Read the model definition and answer for the solid it produces. Units are mm, in the model's axes. A direction names the side the tool comes from. Coordinates: 2 decimals unless noted, no trailing zeros. Order: outer loops, then holes, each group sorted by start corner. A loop starts at its lowest first (then second) coordinate and runs counter-clockwise, first axis right, second up. Notation, with made-up numbers: M 56,68.25 L 75,68.25 A20 ccw 75,88.25 Z; hole C 80.25,87.25 d9. An arc over 180 degrees is marked long. Put each result on its own line as item: value.
from build123d import *

# Parameters (mm, degrees)
CUT_EXTRUDE1_REACH = 68.227
SKETCH4_W          = 8
SKETCH4_H          = 13


with BuildPart() as part:
    # Sketch1 → Revolve1 (revolve)
    with BuildSketch(Plane.XY, mode=Mode.PRIVATE) as revolve1_sk:
        Polygon((0, 25), (0, 7.5), (-40, 7.5), (-40, 6.5), (19, 6.5), (19, 12), (56, 12), (56, 14), (6, 14), (6, 25), align=None)
    revolve(revolve1_sk.sketch.rotate(Axis((-64.900117457, 0, 0), (1, 0, 0)), 180), axis=Axis((-64.900117457, 0, 0), (1, 0, 0)))

    # Sketch4 → Cut-Extrude1 (cut, up to next)
    with BuildSketch(Plane(origin=(0, 0, 0), x_dir=(1, 0, 0), z_dir=(0, 1, 0)), mode=Mode.PRIVATE) as cut_extrude1_sk1:
        with Locations((15, 0)):
            Rectangle(SKETCH4_W, SKETCH4_H)
    cut_extrude1_tool1 = extrude(cut_extrude1_sk1.sketch, amount=-CUT_EXTRUDE1_REACH, mode=Mode.PRIVATE) & part.part
    add(cut_extrude1_tool1.solids().sort_by_distance((15, 0, 0))[0], mode=Mode.SUBTRACT)


solid = part.part
Q1. Find section C-C on y = -2.5. Write down the section's boundary in (x, z).
Answers below:
outline: M -40,-7.07 L 0,-7.07 L 0,-24.87 L 6,-24.87 L 6,-13.77 L 56,-13.77 L 56,-11.74 L 19,-11.74 L 19,-6.5 L 11,-6.5 L 11,-6 L -40,-6 Z; M -40,6 L 11,6 L 11,6.5 L 19,6.5 L 19,11.74 L 56,11.74 L 56,13.77 L 6,13.77 L 6,24.87 L 0,24.87 L 0,7.07 L -40,7.07 Z
Q2. A tool of negligible diameter and unlimited length cuts with its end or side. For faces 5 (the face through (0, -5, -6)), 6 (the face through (11, -10, 0)), 7 (the face through (-40, 6, -3)), 8 (the face through (30.65, 13.986, -0.616)), from which of +Z, -Z, +X, -X, +Y, -Y can it reach the whole face along a straight path? Write none if from no direction.
Answers below:
face 5: -X
face 6: -Y
face 7: +Z, -Z, -X, +Y, -Y
face 8: +X
Q3. Find section D-D on z = 13. Write down the section's boundary in (x, y).
Answers below:
outline: M 0,-21.35 L 6,-21.35 L 6,-5.2 L 56,-5.2 L 56,5.2 L 6,5.2 L 6,21.35 L 0,21.35 Z
Q4. Given pin 1 (6 mm diameter, centred on x = 0.5, z = -12.5, fed in from +Y); pin 2 (1.5 mm diameter, centred on x = -28, y = -4.5, fed in from -Z); pin 3 (4 mm diameter, centred on y = -8.5, z = -1.5, fed in from +X); pin 4 (8 mm diameter, centred on y = 0, z = 0, fed in from +X), each flat-ended and moving along its own axis, determine where each tip first touches the part or whether it passes through.
Answers below:
pin 1: stops at y = 23.12
pin 2: stops at z = -6.5
pin 3: stops at x = 11
pin 4: passes through
Q5. Find section A-A on z = 0. Write down the section's boundary in (x, y), plus the area to 3 significant figures.
Answers below:
outline: M -40,-7.5 L 0,-7.5 L 0,-25 L 6,-25 L 6,-14 L 11,-14 L 11,-6.5 L -40,-6.5 Z; M -40,6.5 L 19,6.5 L 19,12 L 56,12 L 56,14 L 6,14 L 6,25 L 0,25 L 0,7.5 L -40,7.5 Z; M 19,-14 L 56,-14 L 56,-12 L 19,-12 Z
area: 585 mm^2
Q6. Find section B-B on x = -31. Write down the section's boundary in (y, z).
Answers below:
outline: C 0,0 d15; hole C 0,0 d13
Q7. For a pull along Y with two mould halves and no side action, classify faces 1 (the face through (19, -12.5, 0.1)), 2 (the face through (37.759, -11.446, -3.604)), 3 (the face through (19, 8, 0)), 4 (the face through (-20.28, -4.032, -6.324)) as +Y half, -Y half, draft (parallel to the pull), parting line (faces both ways), or undercut.
Answers below:
face 1: draft
face 2: undercut
face 3: undercut
face 4: parting line
Q8. Consider line 1 along Z through (x, y) = (-1.5, 0); line 2 along Z through (x, y) = (33, 0); line 3 along X through (y, z) = (-18, -8.5). Determine where each line is inside the solid, lowest interval first.
Answers below:
line 1: z = -7.5 to -6.5, 6.5 to 7.5
line 2: z = -14 to -12, 12 to 14
line 3: x = 0 to 6
